CAD build for the part. Positions are in the model's coordinates, mm. Coordinates: 2 decimals unless noted, no trailing zeros. Loops run counter-clockwise (first coordinate to the right, second up) from the corner with the lowest first, then second, coordinate; pieces in that order, holes last. Notation, with made-up numbers: (20.5, -26) - (45.5, -26) arc R23 ccw to (45.5, 12) - close; hole circle Ø4 at (80.5, 33.5). An arc over 180 degrees is marked (long way). Put each result on its own line as item: value.
Autodesk Inventor part; units mm, degrees
ref_plane "YZ Plane" through (0, 0, 0) normal (1, 0, 0) x (0, 1, 0)
ref_plane "XZ Plane" through (0, 0, 0) normal (0, 1, 0) x (-1, 0, 0)
ref_plane "XY Plane" through (0, 0, 0) normal (0, 0, 1) x (1, 0, 0)
sketch "Sketch1" plane through (0, 0, 0) normal (1, 0, 0) x (0, 1, 0)
  line L0 (0, -88.9) -> (0, 88.9) construction
  line L1 (-142.24, 0) -> (142.24, 0) construction
  line L2 (101.6, 63.5) -> (-101.6, 63.5)
  line L3 (-101.6, 63.5) -> (-101.6, -63.5)
  line L4 (-101.6, -63.5) -> (101.6, -63.5)
  line L5 (101.6, -63.5) -> (101.6, 63.5)
  point P0 (0, 0)
  point P1 (0, 63.5)
  point P2 (101.6, 0)
  dimension "d0" = 203.2
  dimension "d1" = 127
extrude "Extrusion1" add sketch "Sketch1" along normal blind 3.175
sketch "Sketch2" plane through (3.175, 0, 0) normal (1, 0, 0) x (0, 0, -1)
  line L0 (88.9, 0) -> (-88.9, 0) construction
  line L1 (0, -142.24) -> (0, 142.24) construction
  line L2 (-38.1, -23.8125) -> (38.1, -23.8125) construction
  line L3 (38.1, -23.8125) -> (38.1, -100.0125) construction
  line L4 (38.1, -100.0125) -> (-38.1, -100.0125) construction
  line L5 (-38.1, -100.0125) -> (-38.1, -23.8125) construction
  line L6 (-26.9875, -34.925) -> (26.9875, -34.925) construction
  line L7 (26.9875, -34.925) -> (26.9875, -88.9) construction
  line L8 (26.9875, -88.9) -> (-26.9875, -88.9) construction
  line L9 (-26.9875, -88.9) -> (-26.9875, -34.925) construction
  line L10 (-38.1, -61.9125) -> (38.1, -61.9125) construction
  circle A0 centre (-26.9875, -34.925) radius 5.5563
  circle A1 centre (26.9875, -34.925) radius 5.5563
  circle A2 centre (-26.9875, -88.9) radius 5.5563
  circle A3 centre (26.9875, -88.9) radius 5.5563
  line L11 (-63.5, -101.6) -> (63.5, -101.6) construction
  circle A4 centre (0, -61.9125) radius 9.525
  point P0 (0, 0)
  point P1 (0, -23.8125)
  point P2 (0, -34.925)
  point P3 (-26.9875, -61.9125)
  dimension "d4" = 76.2
  dimension "d5" = 53.975
  dimension "d6" = 11.1125
  dimension "d8" = 19.05
  dimension "d29" = 12.7
extrude "Extrusion2" cut sketch "Sketch2" against normal through all
sketch "Sketch4" plane through (3.175, 0, 0) normal (1, 0, 0) x (0, 0, -1)
  line L0 (88.9, 0) -> (-88.9, 0) construction
  line L1 (0, -144.4625) -> (0, 144.4625) construction
  line L2 (-63.5, 101.6) -> (-38.1, 101.6) construction
  line L3 (-38.1, 101.6) -> (-38.1, -101.6) construction
  line L4 (-38.1, -101.6) -> (-63.5, -101.6) construction
  line L5 (-63.5, -101.6) -> (-63.5, 101.6) construction
  line L6 (-50.8, 101.6) -> (-50.8, -101.6) construction
  line L7 (-38.1, 76.2) -> (-63.5, 76.2) construction
  line L8 (-38.1, 88.9) -> (-63.5, 88.9) construction
  circle A0 centre (-50.8, 88.9) radius 3.175
  circle A1 centre (-50.8, 0) radius 3.175
  circle A2 centre (-50.8, -88.9) radius 3.175
  circle A3 centre (50.8, 88.9) radius 3.175
  circle A4 centre (50.8, 0) radius 3.175
  circle A5 centre (50.8, -88.9) radius 3.175
  point P0 (0, 0)
  dimension "d30" = 25.4
  dimension "d31" = 25.4
  dimension "d32" = 6.35
extrude "Extrusion4" cut sketch "Sketch4" against normal through all
properties part number "Lateral Plate" material "Aluminum 6061"
Q1. Slice it at B-B, the plane z = 0. Give the cut face in (x, y) (1 decimal).
Determined:
outline: (0, -101.6) - (3.2, -101.6) - (3.2, -71.4) - (0, -71.4) - close; (0, -52.4) - (3.2, -52.4) - (3.2, 101.6) - (0, 101.6) - close
Q2. Slice it at A-A, the plane z = -50.8. Give the cut face in (x, y) (3 decimals), then the cut area to 3 significant figures.
Determined:
outline: (0, -101.6) - (3.175, -101.6) - (3.175, -92.075) - (0, -92.075) - close; (0, -85.725) - (3.175, -85.725) - (3.175, -3.175) - (0, -3.175) - close; (0, 3.175) - (3.175, 3.175) - (3.175, 85.725) - (0, 85.725) - close; (0, 92.075) - (3.175, 92.075) - (3.175, 101.6) - (0, 101.6) - close
area: 585 mm2
Q3. Mould opens along Y. For faces 1 (the flat face through (3.175, -1, 1)), 2 (the cylindrical face through (1.61, -86.754, 53.14)), 3 (the cylindrical face through (1.61, -87.95, -53.83)) say: +Y half, -Y half, draft (parallel to the pull), parting line (faces both ways), or undercut.
Determined:
face 1: draft
face 2: undercut
face 3: undercut
Q4. Wall check: L1, parallel to Y at x = 1.9, z = 50.8 (3 decimals); L2, parallel to Y at x = 1.15, z = 22; L3, parallel to Y at x = 1.1, z = 0. Give the ranges that are in metal, low to high. Write a range as from..to.
Determined:
L1: -101.6..-92.075, -85.725..-3.175, 3.175..85.725, 92.075..101.6
L2: -101.6..-91.35, -86.45..-37.37, -32.48..101.6
L3: -101.6..-71.44, -52.39..101.6
Q5. Slice it at D-D, the plane z = -29.5. Give the cut face in (x, y) (3 decimals), then the cut area to 3 significant figures.
Determined:
outline: (0, -101.6) - (3.175, -101.6) - (3.175, -93.856) - (0, -93.856) - close; (0, -83.944) - (3.175, -83.944) - (3.175, -39.881) - (0, -39.881) - close; (0, -29.969) - (3.175, -29.969) - (3.175, 101.6) - (0, 101.6) - close
area: 582 mm2
Q6. Slice it at C-C, the plane y = 88.9. Give the cut face in (x, z) (3 decimals), then the cut area to 3 significant figures.
Determined:
outline: (0, -63.5) - (3.175, -63.5) - (3.175, -53.975) - (0, -53.975) - close; (0, -47.625) - (3.175, -47.625) - (3.175, 47.625) - (0, 47.625) - close; (0, 53.975) - (3.175, 53.975) - (3.175, 63.5) - (0, 63.5) - close
area: 363 mm2
